Check sheet for the drawn part. Datum: minimum x, y, z corner. Units: mm. A direction names the side the tool comes from. Round coordinates to 2 decimals unless told otherwise and drop trailing zeros. Order: outer loops, then holes, each group sorted by start corner. A loop starts at its lowest first (then second) coordinate and runs counter-clockwise, first axis right, second up.
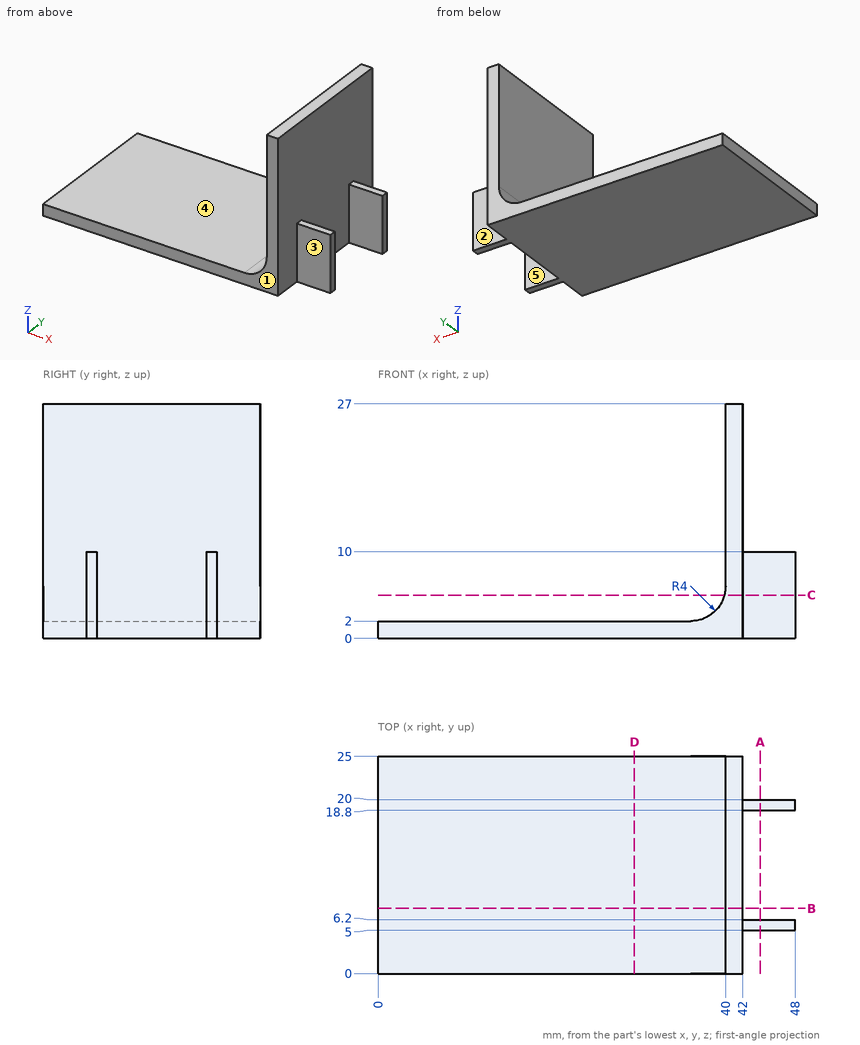
(1) Sectioned sample at A-A, the plane x = 44. Record the cut outline in (y, z), and give its area (3 significant figures).
Returned:
outline: (5, 0) - (6.2, 0) - (6.2, 10) - (5, 10) - close; (18.8, 0) - (20, 0) - (20, 10) - (18.8, 10) - close
area: 24.0 mm2
(2) Depth check by flat-ended pin: P1, Ø3, axis at x = 44.5, z = 7.5, coming from the -Y side; P2, Ø2, axis at y = 14.5, z = 11.5, coming from the +X side; P3, Ø1, axis at x = 44, y = 19.5, coming from the +Z side. Enter the tip coordinate at first touch or a pass-through.
Returned:
P1: stops at y = 5
P2: stops at x = 42
P3: stops at z = 10
(3) Sectioned sample at C-C, the plane z = 5. Record the cut outline in (x, y).
Returned:
outline: (39.87, 0) - (42, 0) - (42, 5) - (48, 5) - (48, 6.2) - (42, 6.2) - (42, 18.8) - (48, 18.8) - (48, 20) - (42, 20) - (42, 25) - (39.87, 25) - close
(4) Sectioned sample at B-B, the plane y = 7.5. Record the cut outline in (x, z).
Returned:
outline: (0, 0) - (42, 0) - (42, 27) - (40, 27) - (40, 6) arc R4 cw to (36, 2) - (0, 2) - close
(5) Set-up check for the marked faces 1, 2, 3, 4 and 5: record each of +Z, -Z, +X, -X, +Y, -Y from which the full face is reachable in a straight line by a thin tool's end or side.
Returned:
face 1: +Z, -Z, +X, -X, -Y
face 2: +Z, -Z, +X, +Y
face 3: +Z, -Z, +X, -Y
face 4: +Z, -X, +Y, -Y
face 5: +Z, -Z, +X
(6) Sectioned sample at D-D, the plane x = 29.5. Record the cut outline in (y, z).
Returned:
outline: (0, 0) - (25, 0) - (25, 2) - (0, 2) - close
(7) Material ranges on line 1 (X direction, y = 16, z = 5.75); line 2 (Z direction, x = 13.5, y = 17.75), recorded low to high.
Returned:
line 1: x = 39.99 to 42
line 2: z = 0 to 2
